Here's how the part is built. I have some questions about the finished solid (model axes, mm). A direction names the side the tool comes from. Round coordinates to 2 decimals unless told otherwise and drop trailing zeros. Write each loop counter-clockwise with the first axis right and the second up, starting at its lowest first coordinate (ties: lowest second). Pieces come first, ordered by that corner, then holes. Notation, with made-up numbers: M 62.25,5 L 72.25,5 A20 ccw 72.25,28 Z; hole C 31,-7 d11. An arc over 180 degrees is marked long. Use one line per item in the form item = value. Start each with the question number.
Q1. I want a section at D-D on x = -45.05. List the corners of the cut face in (y, z) for me.
Q2. I want a section at B-B on z = 42.35. List the corners of the cut face in (x, y) for me (3 decimals).
Q3. I want a section at A-A on x = -46. List the corners of the cut face in (y, z) for me.
Q4. For faces 1 (the face through (-45, 0, 41)), 2 (the face through (-42.86, 0.51, 42.61)), which set-ups out of +Z, -Z, +X, -X, +Y, -Y let a thin tool reach every point of the face, with its end or its side?
Q5. I want a section at C-C on y = -16.5. List the corners of the cut face in (x, z) for me, and give its area (3 significant figures).
Q6. I need wall thicknesses on line 1 along Y through (x, z) = (-43.1, 42.4); line 2 along Y through (x, z) = (-45.7, 42.95); line 3 along X through (y, z) = (-13.25, 42.45). Which ranges of each line are inside material? Lowest first, please. Write a range as from..to.
Q7. I'm going to push flat-ended pins straight in: pin 1 Ø1 at (y, z) = (-15, 43.5) entering from +X; pin 2 Ø1 at (x, y) = (-46, -5.5) entering from +Z; pin 3 Ø1 at (x, y) = (-46.5, -5) entering from +Z. Where does each tip first touch, or does it pass through?
```python
from build123d import *

# Parameters (mm, degrees)
F0_R     = 1.27
F1_DEPTH = 17.78
F2_R     = 2.0534537801
F3_DEPTH = 1.0414
F5_DEPTH = 0.5588


with BuildPart() as f1:
    # F0 (on Front) → F1 (new body)
    with BuildSketch(Plane.XZ):
        with Locations((-44.9135862291, 42.5175279379)):
            Circle(F0_R)
    extrude(amount=F1_DEPTH)

    # F2 (on face) → F3 (join)
    with BuildSketch(Plane(origin=(0, 0, 0), x_dir=(-1, 0, 0), z_dir=(0, 1, 0))):
        with Locations((44.9116155505, 42.5175279379)):
            Circle(F2_R)
        with BuildLine():
            ThreePointArc((44.2763268948, 41.4189832001), (43.6435862291, 42.5175279379), (44.2763268948, 43.6160726756))
            ThreePointArc((44.2763268948, 43.6160726756), (44.9113103393, 43.7875258986), (45.5469042063, 43.6183496036))
            ThreePointArc((45.5469042063, 43.6183496036), (46.0129528265, 43.1533683931), (46.1835862291, 42.5175279379))
            ThreePointArc((46.1835862291, 42.5175279379), (45.5474555553, 41.4170236547), (44.2763268948, 41.4189832001))
        make_face(mode=Mode.SUBTRACT)
        Polygon((44.2763268948, 43.6160726756), (44.2763268948, 42.5175279379), (44.2763268948, 41.4189832001), (45.5469042063, 41.4189832001), (45.5469042063, 43.6183496036), align=None)
        with BuildLine():
            Line((45.5469042063, 41.4189832001), (44.2763268948, 41.4189832001))
            ThreePointArc((44.2763268948, 41.4189832001), (45.5474555553, 41.4170236547), (46.1835862291, 42.5175279379))
            ThreePointArc((46.1835862291, 42.5175279379), (46.0129528265, 43.1533683931), (45.5469042063, 43.6183496036))
            Line((45.5469042063, 43.6183496036), (45.5469042063, 41.4189832001))
        make_face()
        with BuildLine():
            Line((44.2763268948, 41.4189832001), (44.2763268948, 42.5175279379))
            Line((44.2763268948, 42.5175279379), (44.2763268948, 43.6160726756))
            ThreePointArc((44.2763268948, 43.6160726756), (43.6435862291, 42.5175279379), (44.2763268948, 41.4189832001))
        make_face()
        with BuildLine():
            ThreePointArc((45.5469042063, 43.6183496036), (44.9113103393, 43.7875258986), (44.2763268948, 43.6160726756))
            Line((44.2763268948, 43.6160726756), (45.5469042063, 43.6183496036))
        make_face()
    extrude(amount=F3_DEPTH)

    # F4 (on face) → F5 (join)
    with BuildSketch(Plane.XZ.offset(17.78)):
        with BuildLine():
            Line((-45.5651804805, 43.6076311126), (-45.5651804805, 42.5175279379))
            Line((-45.5651804805, 42.5175279379), (-45.5651804805, 41.4274247632))
            ThreePointArc((-45.5651804805, 41.4274247632), (-44.2869382814, 41.4128957142), (-43.6435862291, 42.5175279379))
            ThreePointArc((-43.6435862291, 42.5175279379), (-44.2869382814, 43.6221601616), (-45.5651804805, 43.6076311126))
        make_face()
    extrude(amount=F5_DEPTH)


solid = f1.part
```
Reported:
q1.outline = M -18.34,41.25 L 0,41.25 L 0,40.47 L 1.04,40.47 L 1.04,44.57 L 0,44.57 L 0,43.78 L -18.34,43.78 Z
q2.outline = M -46.958,0 L -46.172,0 L -46.172,-17.78 L -45.565,-17.78 L -45.565,-18.339 L -43.655,-18.339 L -43.655,0 L -42.865,0 L -42.865,1.041 L -46.958,1.041 Z
q3.outline = M -17.78,41.86 L 0,41.86 L 0,40.78 L 1.04,40.78 L 1.04,44.26 L 0,44.26 L 0,43.18 L -17.78,43.18 Z
q4.face_1 = -Y
q4.face_2 = +Y, -Y
q5.outline = C -44.91,42.52 d2.54
q5.area = 5.07 mm^2
q6.line_1 = 0..1.04
q6.line_2 = -17.78..1.04
q6.line_3 = -46.18..-43.65
q7.pin_1 = -43.74
q7.pin_2 = 43.64
q7.pin_3 = 43.18
